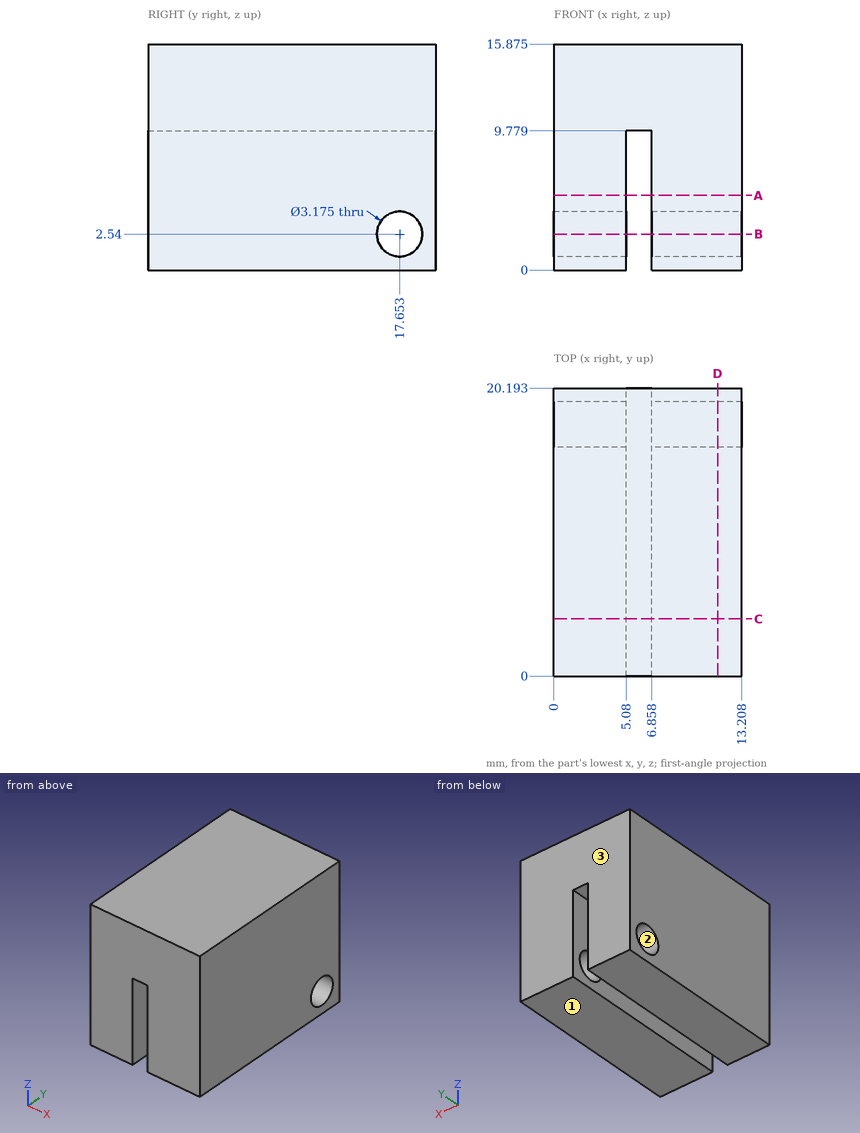
Can you work these out from the drawing? Everything is in mm from the part's minimum corner. Coordinates: 2 decimals unless noted, no trailing zeros. Write each loop counter-clockwise with the first axis right and the second up, starting at its lowest first coordinate (ties: lowest second). Pieces come first, ordered by that corner, then holes. Notation, with made-up numbers: (81, 11.25) -> (107, 11.25) arc R20 cw to (107, 39.25) -> close; hole circle Ø8 at (74, -23). An arc over 180 degrees is marked (long way). Write each question's results on one line, items separated by ' | '. Start each with the question number.
Item 1: Please list where these lines run through material, in increasing order: probe 1 along X at (y, z) = (16.5, 6.5); probe 2 along Y at (x, z) = (9.5, 2.54); probe 3 along Y at (x, z) = (1.5, 1.75).
Item 2: If we section it at B-B, the plane z = 2.54: Write out the boundary of the cut face in (x, y), and give its area (3 significant figures).
Item 3: If we section it at C-C, the plane y = 4: Write out the boundary of the cut face in (x, z) (3 decimals).
Item 4: Thinking about a two-plate mould opening in Y: for the marked faces 1, 2 and 3, which applies, released by +Y, released by -Y, zero draft, split by the parting line, or undercut?
Item 5: If we section it at A-A, the plane z = 5.25: Write out the boundary of the cut face in (x, y).
Item 6: I'm going to push flat-ended pins straight in: P1, Ø2.5, axis at y = 17.653, z = 2.54, coming from the +X side; P2, Ø8, axis at y = 14, z = 13.5, coming from the -X side. Where does each tip first touch, or does it pass through?
Item 7: If we section it at D-D, the plane x = 11.5: Write out the boundary of the cut face in (y, z) (1 decimal).
Answer block:
1) probe 1: 0 to 5.08, 6.86 to 13.21 | probe 2: 0 to 16.07, 19.24 to 20.19 | probe 3: 0 to 16.28, 19.03 to 20.19
2) outline: (0, 0) -> (5.08, 0) -> (5.08, 16.07) -> (0, 16.07) -> close; (0, 19.24) -> (5.08, 19.24) -> (5.08, 20.19) -> (0, 20.19) -> close; (6.86, 0) -> (13.21, 0) -> (13.21, 16.07) -> (6.86, 16.07) -> close; (6.86, 19.24) -> (13.21, 19.24) -> (13.21, 20.19) -> (6.86, 20.19) -> close | area: 195 mm²
3) outline: (0, 0) -> (5.08, 0) -> (5.08, 9.779) -> (6.858, 9.779) -> (6.858, 0) -> (13.208, 0) -> (13.208, 15.875) -> (0, 15.875) -> close
4) face 1: zero draft | face 2: undercut | face 3: released by +Y
5) outline: (0, 0) -> (5.08, 0) -> (5.08, 20.19) -> (0, 20.19) -> close; (6.86, 0) -> (13.21, 0) -> (13.21, 20.19) -> (6.86, 20.19) -> close
6) P1: through | P2: x = 0
7) outline: (0, 0) -> (20.2, 0) -> (20.2, 15.9) -> (0, 15.9) -> close; hole circle Ø3.2 at (17.7, 2.5)
